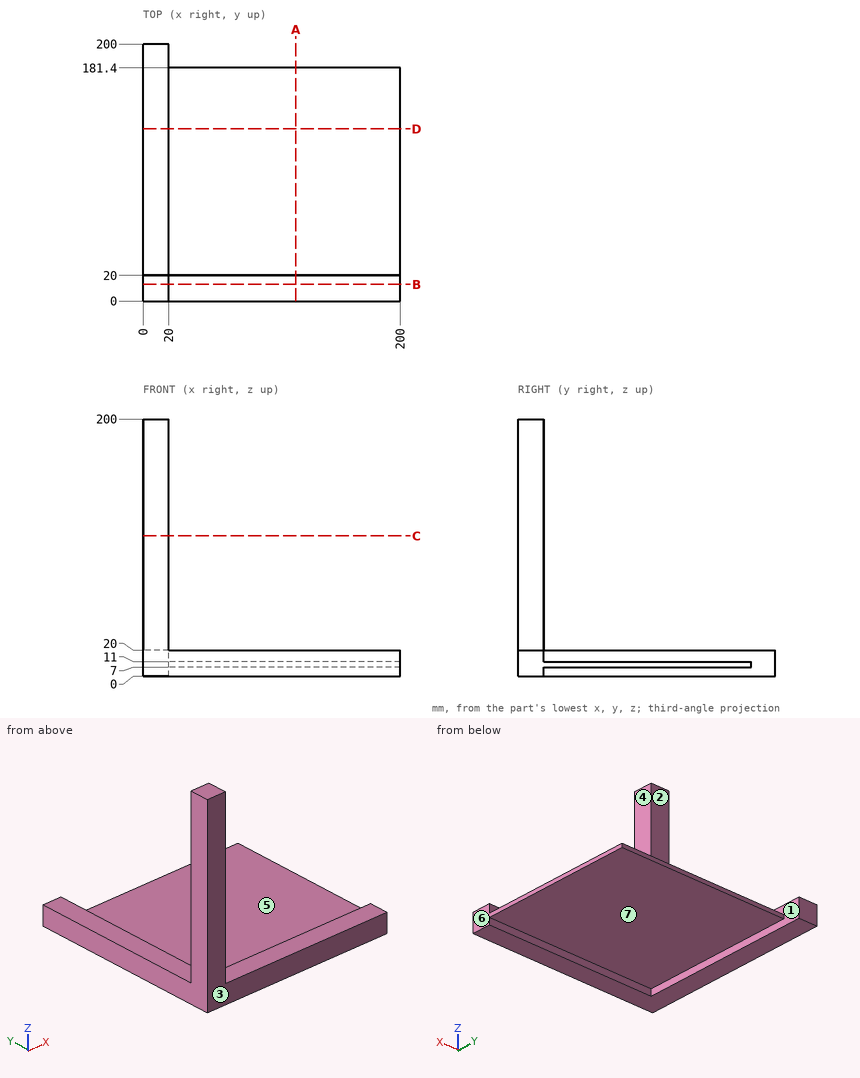
Study the drawing (mm; zero at the part's minimum x, y, z) and answer. A direction names the side the tool comes from. Coordinates: 2 decimals unless noted, no trailing zeros. Write each loop counter-clockwise with the first axis right and the second up, starting at its lowest first coordinate (ties: lowest second). Pieces come first, ordered by that corner, then holes. Notation, with made-up numbers: (-30.75, 29.25) -> (-12.75, 29.25) arc R19 cw to (-12.75, 33.25) -> close; hole circle Ø11 at (17.25, 59). An arc over 180 degrees is marked (long way). Write each question's results on one line, items separated by ' | '. Start each with the question number.
1) A cutting plane is placed at A-A (x = 119). Determine the outline of the cut face in (y, z).
2) A cutting plane is placed at D-D (y = 134). Determine the outline of the cut face in (x, z), then the cut area to 3 significant figures.
3) A tool of negligible diameter and unlimited length cuts with its end or side. For the marked faces 4, 5, 6 and 7, from which of +Z, -Z, +X, -X, +Y, -Y can it reach the whole face along a straight path? Write none if from no direction.
4) A cutting plane is placed at B-B (y = 13). Determine the outline of the cut face in (x, z).
5) A cutting plane is placed at C-C (z = 109). Determine the outline of the cut face in (x, y).
6) For a pull along Y with two mould halves and no side action, classify the marked faces 1, 2 and 3 as +Y half, -Y half, draft (parallel to the pull), parting line (faces both ways), or undercut.
7) Straight lines are drawn through the part: probe 1 along Z at (x, y) = (111.5, 32); probe 2 along X at (y, z) = (62, 18.5). For each, find the intervals that lie inside material, in ascending order.
8) Flat-ended cylindrical pins translate along their axes: pin 1 Ø6 at (x, y) = (106, 11.5) entering from +Z; pin 2 Ø6 at (x, z) = (14, 76) entering from +Y; pin 3 Ø1.2 at (x, z) = (72.5, 10) entering from +Y. Find the tip coordinate at first contact, or state that the pin passes through.
Values follow:
1) outline: (0, 0) -> (20, 0) -> (20, 7) -> (181.4, 7) -> (181.4, 11) -> (20, 11) -> (20, 20) -> (0, 20) -> close
2) outline: (0, 0) -> (20, 0) -> (20, 7) -> (200, 7) -> (200, 11) -> (20, 11) -> (20, 20) -> (0, 20) -> close | area: 1,120 mm²
3) face 4: +Z, +X, +Y, -Y | face 5: +Z, +X, +Y | face 6: +Z, -Z, +X, +Y, -Y | face 7: -Z, +X, +Y
4) outline: (0, 0) -> (200, 0) -> (200, 20) -> (20, 20) -> (20, 200) -> (0, 200) -> close
5) outline: (0, 0) -> (20, 0) -> (20, 20) -> (0, 20) -> close
6) face 1: draft | face 2: +Y half | face 3: -Y half
7) probe 1: 7 to 11 | probe 2: 0 to 20
8) pin 1: z = 20 | pin 2: y = 20 | pin 3: y = 181.4
